from build123d import *

# Parameters (mm, degrees)
F1_DEPTH = 12.7
F2_R     = 2.54


with BuildPart() as f1:
    # F0 (on Top) → F1 (new body)
    with BuildSketch(Plane.XY):
        with BuildLine():
            Line((0, 30.729745), (0, 0))
            Line((0, 0), (33.628508, 0))
            Line((33.628508, 0), (33.628508, 18.006372))
            Line((33.628508, 18.006372), (22.609146, 18.006372))
            ThreePointArc((22.609146, 18.006372), (18.119018, 19.866244), (16.259146, 24.356372))
            Line((16.259146, 24.356372), (16.259146, 30.729745))
            ThreePointArc((16.259146, 30.729745), (14.399274, 35.219873), (9.909146, 37.079745))
            Line((9.909146, 37.079745), (6.35, 37.079745))
            ThreePointArc((6.35, 37.079745), (1.859872, 35.219873), (0, 30.729745))
        make_face()
    extrude(amount=F1_DEPTH)

    # F2
    f2_edges = [f1.edges().sort_by_distance(p)[0] for p in [
        (1.859872, 35.219873, 12.7),
        (8.129573, 37.079745, 12.7),
        (14.399274, 35.219873, 12.7),
        (16.259146, 27.543059, 12.7),
        (18.119018, 19.866244, 12.7),
        (28.118827, 18.006372, 12.7),
        (33.628508, 9.003186, 12.7),
        (16.814254, 0, 12.7),
        (0, 15.364872, 12.7),
    ]]
    fillet(f2_edges, radius=F2_R)


solid = f1.part
Here's how the part is built. I have some questions about the finished solid (model axes, mm). A direction names the side the tool comes from. Round coordinates to 2 decimals unless told otherwise and drop trailing zeros. Loops run counter-clockwise (first coordinate to the right, second up) from the corner with the lowest first, then second, coordinate; pieces in that order, holes last. Notation, with made-up numbers: M -3,-7 L 11,-7 A29 ccw 11,21 Z; hole C 42,-7.75 d7. An arc over 180 degrees is marked long. Write each question's results on one line, items separated by ' | '. Start each with the question number.
(1) If I drill on probe 1 along Y at (x, z) = (6, 4.25); probe 2 along Y at (x, z) = (30.5, 7); probe 3 along X at (y, z) = (28.5, 2.25), over which ranges is the centre line in solid material (lowest first)? Write a range as from..to.
(2) I want a section at B-B (y = 29.5). Please give me the cut outline in (x, z), then the cut area to 3 significant figures.
(3) On a 3-axis mill with a long thin cutter (end or side, diameter ignored), from which of +Z, -Z, +X, -X, +Y, -Y can I reach the whole of each face in a straight line? I mean faces 1 (the flat face through (16.259, 27, 5)), 2 (the cylindrical face through (28.04, 17.28, 11.94)), 3 (the cylindrical face through (32.9, 9.13, 11.94)). Say none if no direction works.
(4) Will these pins go through, and if not, where does the flat tip stop? P1, Ø5, axis at x = 18, y = 21.5, coming from the -Z side; P2, Ø3, axis at x = 19, y = 29, coming from the -Z side; P3, Ø7, axis at y = 27.5, z = 3.5, coming from the +X side.
(5) I want a section at A-A (z = 8). Please give me the cut outline in (x, y).
(6) I want a section at C-C (z = 11.75). Please give me the cut outline in (x, y), then the cut area to 3 significant figures.
Solved:
1) probe 1: y = 0..37.07 | probe 2: y = 0..18.01 | probe 3: x = 0..16.26
2) outline: M 0,0 L 16.26,0 L 16.26,10.16 A2.54 ccw 13.72,12.7 L 2.54,12.7 A2.54 ccw 0,10.16 Z | area: 204 mm²
3) face 1: +Z, -Z, +X, +Y | face 2: +Z, +X, +Y | face 3: +Z, +X, +Y, -Y
4) P1: stops at z = 0 | P2: passes through | P3: stops at x = 16.27
5) outline: M 0,0 L 33.63,0 L 33.63,18.01 L 22.61,18.01 A6.35 cw 16.26,24.36 L 16.26,30.73 A6.35 ccw 9.91,37.08 L 6.35,37.08 A6.35 ccw 0,30.73 Z
6) outline: M 0.56,0.56 L 33.07,0.56 L 33.07,17.45 L 22.61,17.45 A6.91 cw 15.7,24.36 L 15.7,30.73 A5.79 ccw 9.91,36.52 L 6.35,36.52 A5.79 ccw 0.56,30.73 Z | area: 834 mm²
